from build123d import *

# Parameters (mm, degrees)
SKETCH1_R           = 1.75
BOSS_EXTRUDE1_DEPTH = 2


with BuildPart() as part:
    # Sketch1 → Boss-Extrude1 (new body)
    with BuildSketch(Plane.XY):
        with BuildLine():
            Line((6.78007207, 2.305908396), (5.344058207, 1.300400663))
            ThreePointArc((5.344058207, 1.300400663), (4.741801382, 0.631408553), (4.493915363, -0.233933141))
            ThreePointArc((4.493915363, -0.233933141), (0, -4.5), (-4.493915363, -0.233933141))
            ThreePointArc((-4.493915363, -0.233933141), (-4.741801382, 0.631408553), (-5.344058207, 1.300400663))
            Line((-5.344058207, 1.300400663), (-6.78007207, 2.305908396))
            ThreePointArc((-6.78007207, 2.305908396), (-7.614702985, 2.643035912), (-8.512640201, 2.580008285))
            ThreePointArc((-8.512640201, 2.580008285), (-14.136868529, 8.186516868), (-6.347604272, 9.733205303))
            ThreePointArc((-6.347604272, 9.733205303), (-5.656224906, 9.192572354), (-4.799950824, 9))
            Line((-4.799950824, 9), (4.799950824, 9))
            ThreePointArc((4.799950824, 9), (5.656224906, 9.192572354), (6.347604272, 9.733205303))
            ThreePointArc((6.347604272, 9.733205303), (14.136868529, 8.186516868), (8.512640201, 2.580008285))
            ThreePointArc((8.512640201, 2.580008285), (7.614702985, 2.643035912), (6.78007207, 2.305908396))
        make_face()
        Circle(SKETCH1_R, mode=Mode.SUBTRACT)
        with Locations((9.829824531, 6.882917236)):
            Circle(SKETCH1_R, mode=Mode.SUBTRACT)
        with Locations(Location((-9.829824531, 6.882917236, 0), (0, 0, 180))):
            Circle(SKETCH1_R, mode=Mode.SUBTRACT)
    extrude(amount=BOSS_EXTRUDE1_DEPTH)


solid = part.part
For this review, take the finished solid that the model builds, in its own axes (mm). A direction names the side the tool comes from. Give positions to 0.01 mm unless a question says otherwise; leave off trailing zeros. Write each loop counter-clockwise with the first axis right and the second up, starting at its lowest first coordinate (ties: lowest second). Pieces come first, ordered by that corner, then holes. Notation, with made-up numbers: (36, -22.75) -> (71, -22.75) arc R23 ccw to (71, 16.25) -> close; hole circle Ø4 at (16, 25). An arc over 180 degrees is marked (long way). Use CSV: the item, a comma, the result in double quotes.
Q1. Take a section at D-D, the plane x = -3.75. Write out the cut boundary in (y, z), then the cut area to 3 significant figures.
Conclusion:
outline,"(-2.49, 0) -> (9, 0) -> (9, 2) -> (-2.49, 2) -> close"
area,"23.0 mm2"
Q2. To check wall thickness, follow probe 1 along X at (y, z) = (6.75, 0.65); probe 2 along X at (y, z) = (8, 0.95); probe 3 along Y at (x, z) = (9, 1.65). State the ranges of each line that lie inside material, in increasing order. Write a range as [from, to].
Conclusion:
probe 1,"[-14.33, -11.57], [-8.08, 8.08], [11.57, 14.33]"
probe 2,"[-14.19, -11.18], [-8.48, 8.48], [11.18, 14.19]"
probe 3,"[2.46, 5.34], [8.42, 11.31]"
Q3. Take a section at A-A, the plane x = 0. Write out the cut boundary in (y, z), then the cut area to 3 significant figures.
Conclusion:
outline,"(-4.5, 0) -> (-1.75, 0) -> (-1.75, 2) -> (-4.5, 2) -> close; (1.75, 0) -> (9, 0) -> (9, 2) -> (1.75, 2) -> close"
area,"20.0 mm2"
Q4. Take a section at C-C, the plane y = -0.5. Write out the cut boundary in (x, z).
Conclusion:
outline,"(-4.47, 0) -> (-1.68, 0) -> (-1.68, 2) -> (-4.47, 2) -> close; (1.68, 0) -> (4.47, 0) -> (4.47, 2) -> (1.68, 2) -> close"
Q5. For P1, Ø3, axis at x = -9.83, y = 6.88, coming from the -Z side; P2, Ø1, axis at x = -0.5, z = 0.5, coming from the +Y side, all flat-tipped, find the tip position at first contact; note any pin that passes through.
Conclusion:
P1,"through"
P2,"y = 9"
Q6. Tool access review of faces 4 (the face through (0, 5, 0)), 5 (the face through (5.65, 9.19, 0.99)): name each direction out of +Z, -Z, +X, -X, +Y, -Y from which nothing blocks a thin tool from reaching the whole face with its end or side.
Conclusion:
face 4,"-Z, +X, -X, +Y, -Y"
face 5,"+Z, -Z, +Y"
Q7. Take a section at B-B, the plane z = 1.7. Write out the cut boundary in (x, y), then the cut area to 3 significant figures.
Conclusion:
outline,"(-8.51, 2.58) arc R2 cw to (-6.78, 2.31) -> (-5.34, 1.3) arc R2 cw to (-4.49, -0.23) arc R4.5 ccw to (4.49, -0.23) arc R2 cw to (5.34, 1.3) -> (6.78, 2.31) arc R2 cw to (8.51, 2.58) arc R4.5 ccw (long way) to (6.35, 9.73) arc R2 cw to (4.8, 9) -> (-4.8, 9) arc R2 cw to (-6.35, 9.73) arc R4.5 ccw (long way) to start; hole circle Ø3.5 at (-9.83, 6.88); hole circle Ø3.5 at (0, 0); hole circle Ø3.5 at (9.83, 6.88)"
area,"235 mm2"
Q8. Mouldability with a two-part tool opening along Y and no side actions: class faces 1 (the face through (6.07, 1.81, 0.99)), 2 (the face through (14.1, 8.3, 1)), 3 (the face through (-8.54, 5.7, 0.99)) as pulls with the +Y half, pulls with the -Y half, needs draft (parallel to the pull), parting line crosses it, or undercut.
Conclusion:
face 1,"pulls with the -Y half"
face 2,"parting line crosses it"
face 3,"undercut"
